```python
from build123d import *

# Parameters (mm, degrees)
SKETCH1_R           = 2.4892
BOSS_EXTRUDE1_DEPTH = 3.175
FILLET1_R           = 4.7625


with BuildPart() as part:
    # Sketch1 → Boss-Extrude1 (new body)
    with BuildSketch(Plane.XY):
        Polygon((-27.051, 31.75), (-27.051, -29.21), (34.925, -29.21), (34.925, -7.62), (-10.795, -7.62), (-10.795, 31.75), align=None)
        with Locations((-19.05, -19.05)):
            Circle(SKETCH1_R, mode=Mode.SUBTRACT)
        with Locations((-19.05, -6.35)):
            Circle(SKETCH1_R, mode=Mode.SUBTRACT)
        with Locations((0, -19.05)):
            Circle(SKETCH1_R, mode=Mode.SUBTRACT)
        with Locations((12.7, -19.05)):
            Circle(SKETCH1_R, mode=Mode.SUBTRACT)
        with Locations((25.4, -19.05)):
            Circle(SKETCH1_R, mode=Mode.SUBTRACT)
        with Locations((-19.05, 6.35)):
            Circle(SKETCH1_R, mode=Mode.SUBTRACT)
        with Locations((-19.05, 19.05)):
            Circle(SKETCH1_R, mode=Mode.SUBTRACT)
        with Locations((-19.05, -19.05)):
            Circle(SKETCH1_R)
    extrude(amount=BOSS_EXTRUDE1_DEPTH)

    # Fillet1
    fillet1_edges = [part.edges().sort_by_distance(p)[0] for p in [
        (-27.051, 31.75, 1.5875),
        (-10.795, 31.75, 1.5875),
        (-10.795, -7.62, 1.5875),
        (34.925, -7.62, 1.5875),
        (34.925, -29.21, 1.5875),
        (-27.051, -29.21, 1.5875),
    ]]
    fillet(fillet1_edges, radius=FILLET1_R)


solid = part.part
```
Verification items for the finished model (mm, model axes). A direction names the side the tool comes from. Round coordinates to 2 decimals unless told otherwise and drop trailing zeros. Loops run counter-clockwise (first coordinate to the right, second up) from the corner with the lowest first, then second, coordinate; pieces in that order, holes last. Notation, with made-up numbers: (-31, -27) -> (-6, -27) arc R19 ccw to (-6, 3) -> close; hole circle Ø11 at (73, 75.25). An arc over 180 degrees is marked (long way). Answer as a JSON object with one key per item and string values.
Q1. Section check D-D (z = 1.5). State how many separate pieces and enclosed holes the cut face has, then the cut area to 3 significant figures.
Data:
{"separate pieces": "1", "enclosed holes": "6", "area": "1,840 mm2"}
Q2. Go/stop test with flat-tipped pins: P1, Ø2, axis at x = -9.5, y = -3, coming from the -Z side; P2, Ø1, axis at x = 4, z = 2.5, coming from the +Y side; P3, Ø1.5, axis at x = -11, z = 2.5, coming from the +Y side; P4, Ø1, axis at y = 11.5, z = 1, coming from the +X side (3 decimals). Record where each tip stops, or that it passes through.
Data:
{"P1": "passes through", "P2": "stops at y = -7.62", "P3": "stops at y = 29.85", "P4": "stops at x = -10.795"}
Q3. Access from +Z, -Z, +X, -X, +Y, -Y to the whole of each face (thin tool, end or side, straight path). Record for faces 5 (the cylindrical face through (-21.537, -6.241, 1.565)), 6 (the flat face through (-10.795, 12, 2)).
Data:
{"face 5": "+Z, -Z", "face 6": "+Z, -Z, +X, +Y"}
Q4. Section check A-A (x = 25.4). Record the boundary of the cut face in (y, z) (3 decimals).
Data:
{"outline": "(-29.21, 0) -> (-21.539, 0) -> (-21.539, 3.175) -> (-29.21, 3.175) -> close; (-16.561, 0) -> (-7.62, 0) -> (-7.62, 3.175) -> (-16.561, 3.175) -> close"}
Q5. Section check C-C (x = -19.05). Record the boundary of the cut face in (y, z) (3 decimals).
Data:
{"outline": "(-29.21, 0) -> (-8.839, 0) -> (-8.839, 3.175) -> (-29.21, 3.175) -> close; (-3.861, 0) -> (3.861, 0) -> (3.861, 3.175) -> (-3.861, 3.175) -> close; (8.839, 0) -> (16.561, 0) -> (16.561, 3.175) -> (8.839, 3.175) -> close; (21.539, 0) -> (31.75, 0) -> (31.75, 3.175) -> (21.539, 3.175) -> close"}
Q6. Section check B-B (y = 19.05). Record the boundary of the cut face in (x, z) (3 decimals).
Data:
{"outline": "(-27.051, 0) -> (-21.539, 0) -> (-21.539, 3.175) -> (-27.051, 3.175) -> close; (-16.561, 0) -> (-10.795, 0) -> (-10.795, 3.175) -> (-16.561, 3.175) -> close"}
Q7. Draft check along Y on faces 1 (the flat face through (4, -29.21, 2)), 2 (the cylindrical face through (-0.32, -16.58, 1.57)), 3 (the flat face through (34.925, -18, 2)), 4 (the flat face through (12, -7.62, 2)). Enter one of: pulls with the +Y half, pulls with the -Y half, needs draft (parallel to the pull), parting line crosses it, or undercut.
Data:
{"face 1": "pulls with the -Y half", "face 2": "undercut", "face 3": "needs draft", "face 4": "pulls with the +Y half"}
Q8. Scan lines: line 1 (Y direction, x = -19, z = 2.7); line 2 (Y direction, x = 12.7, z = 0.75); line 3 (Y direction, x = -21, z = 2.7). Record each from-to range of solid material in increasing order. Write a range as from..to.
Data:
{"line 1": "y = -29.21..-8.84, -3.86..3.86, 8.84..16.56, 21.54..31.75", "line 2": "y = -29.21..-21.54, -16.56..-7.62", "line 3": "y = -29.21..-7.9, -4.8..4.8, 7.9..17.5, 20.6..31.75"}
